```python
from build123d import *

# Parameters (mm, degrees)
SKETCH_1_R      = 1.5
SKETCH_1_R_2    = 14
SKETCH_1_R_3    = 2.6
EXTRUDE_1_DEPTH = 3


with BuildPart() as part:
    # 草图1 → 凸台-拉伸1 (new body)
    with BuildSketch(Plane(origin=(0, 0, 0), x_dir=(1, 0, 0), z_dir=(0, 1, 0))):
        Polygon((-60, 10), (-20, 10), (-7, 23), (7, 23), (20, 10), (20, -10), (7, -23), (-7, -23), (-20, -10), (-60, -10), align=None)
        with Locations((-35, 6)):
            Circle(SKETCH_1_R, mode=Mode.SUBTRACT)
        with Locations((-50, 6)):
            Circle(SKETCH_1_R, mode=Mode.SUBTRACT)
        with Locations((-35, -6)):
            Circle(SKETCH_1_R, mode=Mode.SUBTRACT)
        with Locations((-50, -6)):
            Circle(SKETCH_1_R, mode=Mode.SUBTRACT)
        Circle(SKETCH_1_R_2, mode=Mode.SUBTRACT)
        with Locations((0, 18)):
            Circle(SKETCH_1_R_3, mode=Mode.SUBTRACT)
        with Locations((0, -18)):
            Circle(SKETCH_1_R_3, mode=Mode.SUBTRACT)
    extrude(amount=EXTRUDE_1_DEPTH)


solid = part.part
```
Geometry: final body of the model. Coordinates: model frame, mm. A direction names the side the tool comes from. Coordinates: 2 decimals unless noted, no trailing zeros. Loops run counter-clockwise (first coordinate to the right, second up) from the corner with the lowest first, then second, coordinate; pieces in that order, holes last. Notation, with made-up numbers: M 86,8 L 108,8 A23 cw 108,41 Z; hole C 64.5,-3.75 d5. An arc over 180 degrees is marked long. Put each result on its own line as item: value.
(1) Draft query along Z for faces 1 (the face through (-0.338, 1.479, -20.578)), 2 (the face through (-13, 1, 17)), 3 (the face through (20, 1, 0)). Return one class per face: pulls with the +Z half, pulls with the -Z half, needs draft (parallel to the pull), parting line crosses it, or undercut.
Answer sheet:
face 1: undercut
face 2: pulls with the +Z half
face 3: needs draft
(2) Cut plane C-C on x = 0. Return the cut outline in (y, z).
Answer sheet:
outline: M 0,-23 L 3,-23 L 3,-20.6 L 0,-20.6 Z; M 0,-15.4 L 3,-15.4 L 3,-14 L 0,-14 Z; M 0,14 L 3,14 L 3,15.4 L 0,15.4 Z; M 0,20.6 L 3,20.6 L 3,23 L 0,23 Z
(3) Cut plane A-A on x = -35. Return the cut outline in (y, z).
Answer sheet:
outline: M 0,-10 L 3,-10 L 3,-7.5 L 0,-7.5 Z; M 0,-4.5 L 3,-4.5 L 3,4.5 L 0,4.5 Z; M 0,7.5 L 3,7.5 L 3,10 L 0,10 Z
(4) Cut plane B-B on z = 0. Return the cut outline in (x, y).
Answer sheet:
outline: M -60,0 L -14,0 L -14,3 L -60,3 Z; M 14,0 L 20,0 L 20,3 L 14,3 Z
(5) Access query for faces 4 (the face through (-40, 1, 10)), 5 (the face through (-19, 3, 0)), 6 (the face through (-40, 1, -10)). Directions: +Z, -Z, +X, -X, +Y, -Y. A direction counts if a zero-diameter tool reaches every point of the face in a straight line with its end or side. Return the directions, or none.
Answer sheet:
face 4: +Z, -X, +Y, -Y
face 5: +Z, -Z, +X, -X, +Y
face 6: -Z, -X, +Y, -Y
(6) Cut plane D-D on y = 1.5. Return the cut outline in (x, z), then the cut area to 3 significant figures.
Answer sheet:
outline: M -60,-10 L -20,-10 L -7,-23 L 7,-23 L 20,-10 L 20,10 L 7,23 L -7,23 L -20,10 L -60,10 Z; hole C -50,-6 d3; hole C -50,6 d3; hole C -35,-6 d3; hole C -35,6 d3; hole C 0,0 d28; hole C 0,-18 d5.2; hole C 0,18 d5.2
area: 1,620 mm^2
(7) First-contact query: pin 1 (1.5 mm diameter, centred on x = -41, y = 1, fed in from +Z); pin 2 (1 mm diameter, centred on x = -19, y = 0.5, fed in from +Z). Flat tips, straight axial feed; report the tip coordinate or a pass-through.
Answer sheet:
pin 1: stops at z = 10
pin 2: stops at z = 11.5
(8) Material intervals for probe 1 along Z at (x, y) = (-35, 0.8); probe 2 along Z at (x, y) = (0, 1.2); probe 3 along X at (y, z) = (1.75, 6), sorted ascending.
Answer sheet:
probe 1: z = -10 to -7.5, -4.5 to 4.5, 7.5 to 10
probe 2: z = -23 to -20.6, -15.4 to -14, 14 to 15.4, 20.6 to 23
probe 3: x = -60 to -51.5, -48.5 to -36.5, -33.5 to -12.65, 12.65 to 20
